```python
from build123d import *
from build123d.topology import SkipClean

# Parameters (mm, degrees)
SKETCH1_W               = 84.00796
SKETCH1_H               = 71.2724
BOSS_EXTRUDE1_DEPTH     = 3.175
SKETCH5_R               = 4.7625
BOSS_EXTRUDE3_DEPTH     = 3.175
SKETCH3_R               = 1.8415
CUT_EXTRUDE1_DEPTH      = 114.886040389
BOSS_EXTRUDE4_START     = 18.542
SKETCH6_R               = 4.7625
BOSS_EXTRUDE4_DEPTH     = 18.542
CUT_EXTRUDE2_DEPTH      = 116.341906237
CUT_EXTRUDE2_DEPTH_BACK = 116.341906237
SKETCH4_R               = 1.778
SKETCH7_R               = 1.778
CUT_EXTRUDE3_DEPTH      = 116.894683482
SKETCH8_R               = 3.556
SKETCH8_R_2             = 3.4925
CUT_EXTRUDE4_DEPTH      = 116.894683482
CUT_EXTRUDE5_DEPTH      = 116.894683482
FILLET1_R               = 3.175
BOSS_EXTRUDE5_DEPTH     = 3.175
CUT_EXTRUDE7_DEPTH      = 5.08


with BuildPart() as part:
    # Sketch1 → Boss-Extrude1 (new body)
    with BuildSketch(Plane.XY):
        with Locations((42.00398, 35.6362)):
            Rectangle(SKETCH1_W, SKETCH1_H)
    extrude(amount=BOSS_EXTRUDE1_DEPTH)

    # Sketch5 → Boss-Extrude3 (add)
    with BuildSketch(Plane.XY.offset(3.175)):
        with Locations((84.00796, 39.524999944)):
            Circle(SKETCH5_R)
        with Locations((0, 39.524999944)):
            Circle(SKETCH5_R)
    extrude(amount=-BOSS_EXTRUDE3_DEPTH)

    # Sketch3 → Cut-Extrude1 (cut, through all)
    with BuildSketch(Plane.XY.offset(3.175)):
        with Locations((42.00398, 4.7625)):
            Circle(SKETCH3_R)
    extrude(amount=-CUT_EXTRUDE1_DEPTH, mode=Mode.SUBTRACT)

    # Sketch6 → Boss-Extrude4 (add)
    with BuildSketch(Plane.XY.offset(3.175).offset(BOSS_EXTRUDE4_START)):
        with Locations((84.00796, 39.524999944)):
            Circle(SKETCH6_R)
        with Locations((0, 39.524999944)):
            Circle(SKETCH6_R)
        with Locations(Location((42.00398, 4.7625, 0), (0, 0, 270))):
            Circle(SKETCH6_R)
        with BuildLine():
            Line((35.65398, 71.2724), (48.35398, 71.2724))
            Line((48.35398, 71.2724), (48.35398, 45.8724))
            ThreePointArc((48.35398, 45.8724), (42.00398, 39.5224), (35.65398, 45.8724))
            Line((35.65398, 45.8724), (35.65398, 71.2724))
        make_face()
    extrude(amount=-BOSS_EXTRUDE4_DEPTH)

    # Sketch4 → Cut-Extrude2 (cut, two sides: drawn at the far end of the back side and taken through both)
    with BuildSketch(Plane.XY.offset(3.175).offset(-CUT_EXTRUDE2_DEPTH_BACK)):
        with Locations((42.00398, 64.9224)):
            Circle(SKETCH4_R)
        with Locations((42.00398, 55.1434)):
            Circle(SKETCH4_R)
        with Locations((42.00398, 45.3644)):
            Circle(SKETCH4_R)
    extrude(amount=CUT_EXTRUDE2_DEPTH + CUT_EXTRUDE2_DEPTH_BACK, mode=Mode.SUBTRACT)

    # Sketch7 → Cut-Extrude3 (cut, through all)
    with BuildSketch(Plane(origin=(0, 0, 0), x_dir=(-1, 0, 0), z_dir=(0, 0, -1))):
        with Locations((-42.00398, 4.7625)):
            Circle(SKETCH7_R)
        with Locations((0, 39.524999944)):
            Circle(SKETCH7_R)
        with Locations((-84.00796, 39.524999944)):
            Circle(SKETCH7_R)
    extrude(amount=-CUT_EXTRUDE3_DEPTH, mode=Mode.SUBTRACT)

    # Sketch8 → Cut-Extrude4 (cut, through all)
    with BuildSketch(Plane(origin=(0, 0, 0), x_dir=(-1, 0, 0), z_dir=(0, 0, -1))):
        with Locations((-61.05398, 24.524999972)):
            Circle(SKETCH8_R)
        with Locations((-22.95398, 24.524999972)):
            Circle(SKETCH8_R_2)
    extrude(amount=-CUT_EXTRUDE4_DEPTH, mode=Mode.SUBTRACT)

    # Sketch9 → Cut-Extrude5 (cut, through all)
    with BuildSketch(Plane(origin=(0, 0, 0), x_dir=(-1, 0, 0), z_dir=(0, 0, -1))):
        Polygon((-84.00796, 0), (-84.00796, 31.587499944), (-45.90796, 0), align=None)
        Polygon((-84.00796, 71.2724), (-84.00796, 47.462499944), (-48.35398, 71.2724), align=None)
    cut_extrude5 = extrude(amount=-CUT_EXTRUDE5_DEPTH, mode=Mode.SUBTRACT)

    # Mirror1: Cut-Extrude5 across plane
    add(cut_extrude5.mirror(Plane(origin=(42.00398, 0, 0), x_dir=(0, 0, 1), z_dir=(1, 0, 0))), mode=Mode.SUBTRACT)

    # Fillet1
    # the kernel refuses this fillet: 3.175 mm, written as the material it adds along each edge
    with BuildSketch(Plane(origin=(84.00796, 34.762499944, 0), x_dir=(0.9789063129307042, 0.2043096436892158, 0), z_dir=(0, 0, 1))) as fillet1_piece_1:
        with BuildLine():
            CenterArc((2.594732475, -3.108027544), FILLET1_R, 101.789089239, 66.421821522)
            Line((-0.513295069, -2.459344425), (0, 0))
            ThreePointArc((0, 0), (0.973024678, -0.100458685), (1.946049356, 0))
        make_face()
    extrude(amount=3.175)
    with BuildSketch(Plane(origin=(84.00796, 44.287499944, 0), x_dir=(0, 1, 0), z_dir=(0, 0, 1)), Plane(origin=(0, 34.762499944, 0), x_dir=(0, -1, 0), z_dir=(0, 0, 1))) as fillet1_piece_2:
        with BuildLine():
            CenterArc((2.512338916, -3.175), FILLET1_R, 90, 66.421821522)
            ThreePointArc((-0.397596651, -1.905), (-0.100458685, -0.973024678), (0, 0))
            Line((0, 0), (2.512338916, 0))
        make_face()
    extrude(amount=3.175)
    with BuildSketch(Plane(origin=(0, 44.287499944, 0), x_dir=(0, 1, 0), z_dir=(0, 0, 1))) as fillet1_piece_3:
        with BuildLine():
            CenterArc((2.512338916, 3.175), FILLET1_R, 203.578178478, 66.421821522)
            ThreePointArc((-0.397596651, 1.905), (-0.100458685, 0.973024678), (0, 0))
            Line((0, 0), (2.512338916, 0))
        make_face()
    extrude(amount=3.175)

    # Sketch10 → Boss-Extrude5 (add)
    with BuildSketch(Plane(origin=(0, 0, 0), x_dir=(-1, 0, 0), z_dir=(0, 0, -1))):
        with BuildLine():
            Line((-23.070402794, 12.460561704), (-28.975644685, 7.564713202))
            ThreePointArc((-28.975644685, 7.564713202), (-13.458086548, 12.356642178), (-5.873921435, 26.717618238))
            Line((-5.873921435, 26.717618238), (-11.078476776, 22.402686701))
            ThreePointArc((-11.078476776, 22.402686701), (-11.084404387, 22.364145909), (-11.091119617, 22.325734519))
            ThreePointArc((-11.091119617, 22.325734519), (-15.284227222, 15.211616198), (-23.070402794, 12.460561704))
        make_face()
    extrude(amount=-BOSS_EXTRUDE5_DEPTH)

    # Sketch11 → Cut-Extrude7 (cut)
    with SkipClean():  # the faces are left unmerged after this step: merging them gives an invalid solid
        with BuildSketch(Plane(origin=(0, 0, 0), x_dir=(-1, 0, 0), z_dir=(0, 0, -1))):
            with BuildLine():
                ThreePointArc((-25.8996445, 32.236555305), (-24.799823539, 34.695913728), (-27.259181962, 35.795734689))
                ThreePointArc((-27.259181962, 35.795734689), (-34.829175406, 22.39334356), (-23.070402794, 12.460561704))
                Line((-23.070402794, 12.460561704), (-11.078476776, 22.402686701))
                ThreePointArc((-11.078476776, 22.402686701), (-11.084404387, 22.364145909), (-11.091119617, 22.325734519))
                ThreePointArc((-11.091119617, 22.325734519), (-10.939621184, 23.420732233), (-10.88898, 24.524999972))
                ThreePointArc((-10.88898, 24.524999972), (-12.79398, 26.429999972), (-14.69898, 24.524999972))
                ThreePointArc((-14.69898, 24.524999972), (-27.635249302, 17.725680688), (-25.8996445, 32.236555305))
            make_face()
            with BuildLine():
                ThreePointArc((-21.368554277, 36.485378322), (-24.356904724, 36.508155951), (-27.259181962, 35.795734689))
                ThreePointArc((-27.259181962, 35.795734689), (-24.799823539, 34.695913728), (-25.8996445, 32.236555305))
                ThreePointArc((-25.8996445, 32.236555305), (-23.913875864, 32.724001431), (-21.869215031, 32.708416738))
                ThreePointArc((-21.869215031, 32.708416738), (-19.730403862, 34.346567153), (-21.368554277, 36.485378322))
            make_face()
        extrude(amount=-CUT_EXTRUDE7_DEPTH, mode=Mode.SUBTRACT)


solid = part.part
```
Check sheet for the modelled part. Datum: model origin and axes. Units: mm. A direction names the side the tool comes from. Round coordinates to 2 decimals unless told otherwise and drop trailing zeros. Order: outer loops, then holes, each group sorted by start corner. A loop starts at its lowest first (then second) coordinate and runs counter-clockwise, first axis right, second up. Notation, with made-up numbers: (27.25, -29) - (63.25, -29) arc R10 cw to (63.25, -17) - close; hole circle Ø4 at (43.5, 83). An arc over 180 degrees is marked (long way). Answer as CSV lines item,"result". Start each with the question number.
1) Section check A-A (z = 6.5). Give the number of separate pieces and of enclosed holes in the cut face, then the cut area to 3 significant figures.
2) Section check D-D (x = 50). Record the cut outline in (y, z) (3 decimals), then the cut area to 3 significant figures.
3) Draft check along Y on faces 4 (the face through (19.736, 34.305, 1.565)), 5 (the face through (86, 40, 21.717)), 6 (the face through (13.64, 12.21, 1.57)), 7 (the face through (40.362, 4.082, 12.316)). Enter one of: +Y half, -Y half, draft (parallel to the pull), parting line (faces both ways), or undercut.
4) Scan lines: probe 1 along Y at (x, z) = (0, 10.25); probe 2 along Z at (x, y) = (50.5, 53.5) (3 decimals); probe 3 along X at (y, z) = (47.5, 13). Record each from-to range of solid material in increasing order.
5) Depth check by flat-ended pin: pin 1 (2 mm diameter, centred on x = 84.01, y = 39.52, fed in from +Z); pin 2 (21.5 mm diameter, centred on x = 63, y = 40, fed in from +Z) (3 decimals); pin 3 (6 mm diameter, centred on y = 52.5, z = 3, fed in from +X); pin 4 (0.7 mm diameter, centred on y = 32, z = 2, fed in from -X). Enter the tip coordinate at first touch or a pass-through.
6) Tool access check on faces 1 (the face through (64.607, 24.681, 1.565)), 2 (the face through (88.463, 41.209, 11.011)), 3 (the face through (35.654, 58, 13)). Record the directions out of +Z, -Z, +X, -X, +Y, -Y that give a thin tool (end or side, any length) a straight path to the whole face; none if there is none.
7) Section check C-C (y = 49.5). Record the cut outline in (x, z) (3 decimals), then the cut area to 3 significant figures.
8) Section check B-B (y = 30.5). Record the cut outline in (x, z) (3 decimals).
Determined:
1,separate pieces,"4"
1,enclosed holes,"6"
1,area,"540 mm^2"
2,outline,"(3.393, 0) - (70.173, 0) - (70.173, 3.175) - (3.393, 3.175) - close"
2,area,"212 mm^2"
3,face 4,"undercut"
3,face 5,"draft"
3,face 6,"-Y half"
3,face 7,"undercut"
4,probe 1,"34.76 to 37.75, 41.3 to 44.29"
4,probe 2,"0 to 3.175"
4,probe 3,"35.65 to 48.35"
5,pin 1,"through"
5,pin 2,"z = 3.175"
5,pin 3,"x = 80.96"
5,pin 4,"x = 0"
6,face 1,"+Z, -Z"
6,face 2,"+Z"
6,face 3,"+Z, -X, +Y, -Y"
7,outline,"(3.051, 0) - (80.957, 0) - (80.957, 3.175) - (48.354, 3.175) - (48.354, 21.717) - (35.654, 21.717) - (35.654, 3.175) - (3.051, 3.175) - close"
7,area,"483 mm^2"
8,outline,"(1.312, 0) - (28.65, 0) - (28.65, 3.175) - (1.312, 3.175) - close; (33.436, 0) - (82.696, 0) - (82.696, 3.175) - (33.436, 3.175) - close"
